Check sheet for the drawn part. Datum: minimum x, y, z corner. Units: mm. A direction names the side the tool comes from. Give positions to 0.01 mm unless a question says otherwise; leave off trailing zeros. Write each loop counter-clockwise with the first axis right and the second up, starting at its lowest first coordinate (ties: lowest second). Pieces come first, ordered by that corner, then holes.
(1) Cross-section at C-C (z = 15.25). Record the boundary of the cut face in (x, y) (1 decimal), and give its area (3 significant figures).
(2) Mould release check, pull along X, two halves, no side actions. Record for the marked faces 4, 5, 6 and 7: +X half, -X half, draft (parallel to the pull), parting line (faces both ways), or undercut.
(3) Cross-section at A-A (z = 6.5). Record the boundary of the cut face in (x, y) (1 decimal).
(4) Tool access check on the marked faces 1, 2 and 3. Record the directions out of +Z, -Z, +X, -X, +Y, -Y that give a thin tool (end or side, any length) a straight path to the whole face; none if there is none.
(5) Cross-section at B-B (x = 14.5). Record the boundary of the cut face in (y, z) (1 decimal).
(6) Thickness scan on line 1 along X through (y, z) = (15.5, 5); line 2 along X through (y, z) = (17.25, 6) (1 decimal); line 3 along Z through (x, y) = (19.25, 17.25) (1 decimal). Record the ranges inside material, lowest first.
(7) Cross-section at D-D (y = 6). Record the boundary of the cut face in (x, z) (1 decimal), and give its area (3 significant figures).
(8) Depth check by flat-ended pin: P1, Ø3.5, axis at x = 9.5, y = 10.5, coming from the +Z side. Enter the tip coordinate at first touch or a pass-through.
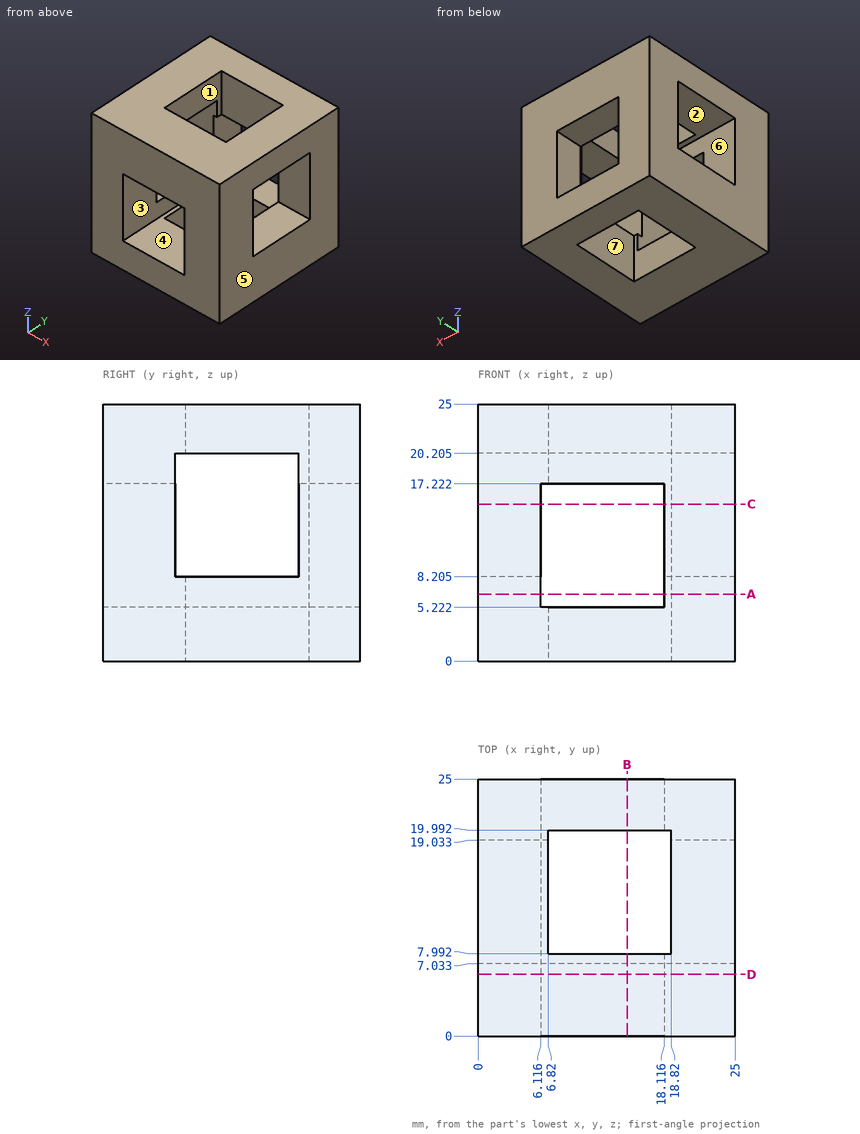
Reply:
1. outline: (0, 0) - (6.1, 0) - (6.1, 7) - (0, 7) - close; (0, 19) - (6.1, 19) - (6.1, 25) - (0, 25) - close; (18.1, 0) - (25, 0) - (25, 7) - (18.1, 7) - close; (18.1, 20) - (18.8, 20) - (18.8, 19) - (25, 19) - (25, 25) - (18.1, 25) - close
1. area: 168 mm2
2. face 4: undercut
2. face 5: +X half
2. face 6: draft
2. face 7: undercut
3. outline: (0, 0) - (6.1, 0) - (6.1, 25) - (0, 25) - close; (18.1, 0) - (25, 0) - (25, 25) - (18.1, 25) - (18.1, 20) - (18.8, 20) - (18.8, 8) - (18.1, 8) - close
4. face 1: +Z, -Z
4. face 2: +X, -X
4. face 3: +Y, -Y
5. outline: (0, 0) - (8, 0) - (8, 5.2) - (0, 5.2) - close; (0, 17.2) - (7, 17.2) - (7, 20.2) - (8, 20.2) - (8, 25) - (0, 25) - close; (20, 0) - (25, 0) - (25, 5.2) - (20, 5.2) - close; (20, 17.2) - (25, 17.2) - (25, 25) - (20, 25) - close
6. line 1: x = 0 to 6.82, 18.82 to 25
6. line 2: x = 0 to 6.1, 18.8 to 25
6. line 3: z = 0 to 8.2, 20.2 to 25
7. outline: (0, 0) - (25, 0) - (25, 25) - (0, 25) - close; hole (6.1, 5.2) - (18.1, 5.2) - (18.1, 17.2) - (6.1, 17.2) - close
7. area: 481 mm2
8. P1: passes through
